Build history of the part. All positions in model axes, mm. A direction names the side the tool comes from. Round coordinates to 2 decimals unless told otherwise and drop trailing zeros. Write each loop counter-clockwise with the first axis right and the second up, starting at its lowest first coordinate (ties: lowest second). Pieces come first, ordered by that corner, then holes.
1) Saw through at C-C (x = 14.5). State how many separate pieces and enclosed holes the cut face has, plus the area to 3 significant figures.
2) Flat gauge pins, fed straight in: pin 1 (5.5 mm diameter, centred on x = 8.5, y = 12.5, fed in from -Z); pin 2 (1 mm diameter, centred on x = 4.5, z = 8, fed in from -Y). Where does each tip first touch, or does it go through?
3) Saw through at A-A (y = 2). Write the cut outline in (x, z) (3 decimals).
4) Pull direction Y, two halves, no side cores. Call faces 3 (the flat face through (19.05, 24, 15)), 4 (the cylindrical face through (9.66, 26.06, 0.45)), 5 (the cylindrical face through (15.097, 11.089, 30.682)), 6 (the cylindrical face through (0.48, 0.45, 1.57)): +Y half, -Y half, draft (parallel to the pull), parting line (faces both ways), or undercut.
5) Wall check: probe 1 along Z at (x, y) = (15.75, 3.75) (3 decimals); probe 2 along X at (y, z) = (13.5, 2); probe 3 along Y at (x, z) = (7.5, 12). Give the ranges that are in metal, low to high.
6) Which spindle directions (+Z, -Z, +X, -X, +Y, -Y) get a long thin tool onto all of the face, cutting with end or side? Do faces 1 (the flat face through (9, 23.367, 16)), 2 (the flat face through (9, 0, 31)). Say none if no direction does.
from build123d import *

# Parameters (mm, degrees)
F1_DEPTH = 19.05
F2_R     = 6.1595
F3_DEPTH = 25.4
F4_R     = 5.842
F5_DEPTH = 3.175
F6_R     = 1.5875
F7_SIZE  = 0.762


with BuildPart() as f1:
    # F0 (on Right) → F1 (new body)
    with BuildSketch(Plane.YZ):
        Polygon((0, 3.175), (0, 0), (26.542, 0), (26.542, 32.258), (0, 32.258), (0, 29.083), (23.367, 29.083), (23.367, 3.175), align=None)
    extrude(amount=F1_DEPTH)

    # F2 (on face) → F3 (cut)
    with BuildSketch(Plane.XY.offset(3.175)):
        with Locations((9.525, 9.3345)):
            Circle(F2_R)
    extrude(amount=-F3_DEPTH, mode=Mode.SUBTRACT)

    # F4 (on face) → F5 (cut, through all)
    with BuildSketch(Plane.XY.offset(32.258)):
        with Locations((9.525, 9.3345)):
            Circle(F4_R)
    extrude(amount=-F5_DEPTH, mode=Mode.SUBTRACT)

    # F6
    f6_edges = [f1.edges().sort_by_distance(p)[0] for p in [
        (19.05, 0, 30.6705),
        (0, 0, 30.6705),
        (0, 0, 1.5875),
        (19.05, 0, 1.5875),
        (9.525, 26.542, 32.258),
        (9.525, 26.542, 0),
    ]]
    fillet(f6_edges, radius=F6_R)

    # F7
    f7_edges = [f1.edges().sort_by_distance(p)[0] for p in [
        (3.3655, 9.3345, 0),
        (3.683, 9.3345, 29.083),
        (3.683, 9.3345, 32.258),
        (3.3655, 9.3345, 3.175),
    ]]
    chamfer(f7_edges, length=F7_SIZE)


solid = f1.part
Evaluation:
1. separate pieces: 3
1. enclosed holes: 0
1. area: 203 mm2
2. pin 1: stops at z = 29.61
2. pin 2: stops at y = 23.37
3. outline: (0, 0) - (19.05, 0) - (19.05, 3.175) - (0, 3.175) - close; (0, 29.083) - (19.05, 29.083) - (19.05, 32.258) - (0, 32.258) - close
4. face 3: draft
4. face 4: +Y half
4. face 5: undercut
4. face 6: -Y half
5. probe 1: z = 0 to 3.175, 29.083 to 32.258
5. probe 2: x = 0 to 4.99, 14.06 to 19.05
5. probe 3: y = 23.37 to 26.54
6. face 1: +X, -X, -Y
6. face 2: +Z, -Z, +X, -X, -Y
